Part model, mm, in its own coordinate system. Face numbers are marked on the shaded views. A direction names the side the tool comes from. Round coordinates to 2 decimals unless told otherwise and drop trailing zeros. Loops run counter-clockwise (first coordinate to the right, second up) from the corner with the lowest first, then second, coordinate; pieces in that order, holes last. Notation, with made-up numbers: (46, 4) - (94, 4) arc R27 cw to (94, 20) - close; hole circle Ø5 at (74, 62). An arc over 180 degrees is marked (long way). Put each result on its own line as item: value.
from build123d import *

# Parameters (mm, degrees)
SKETCH3_R               = 9
EXTRUDE2_DEPTH          = 28.5
EXTRUDE2_DEPTH_BACK     = 28.5
SKETCH4_R               = 9
SKETCH4_R_2             = 7.8
CUT_EXTRUDE2_DEPTH      = 26.5
CUT_EXTRUDE2_DEPTH_BACK = 26.5
SKETCH5_R               = 3.5
EXTRUDE3_DEPTH          = 48.5
EXTRUDE3_DEPTH_BACK     = 48.5


with BuildPart() as part:
    # Sketch3 → Extrude2 (new body, two sides)
    with BuildSketch(Plane(origin=(0, 0, 0), x_dir=(1, 0, 0), z_dir=(0, 1, 0))) as extrude2_sk:
        Circle(SKETCH3_R)
    extrude(amount=EXTRUDE2_DEPTH)
    extrude(extrude2_sk.sketch, amount=-EXTRUDE2_DEPTH_BACK)

    # Sketch4 → Cut-Extrude2 (cut, two sides)
    with BuildSketch(Plane(origin=(0, 0, 0), x_dir=(1, 0, 0), z_dir=(0, 1, 0))) as cut_extrude2_sk:
        Circle(SKETCH4_R)
        Circle(SKETCH4_R_2, mode=Mode.SUBTRACT)
    extrude(amount=CUT_EXTRUDE2_DEPTH, mode=Mode.SUBTRACT)
    extrude(cut_extrude2_sk.sketch, amount=-CUT_EXTRUDE2_DEPTH_BACK, mode=Mode.SUBTRACT)

    # Sketch5 → Extrude3 (add, two sides)
    with BuildSketch(Plane(origin=(0, 0, 0), x_dir=(1, 0, 0), z_dir=(0, 1, 0))) as extrude3_sk:
        Circle(SKETCH5_R)
    extrude(amount=EXTRUDE3_DEPTH)
    extrude(extrude3_sk.sketch, amount=-EXTRUDE3_DEPTH_BACK)


solid = part.part
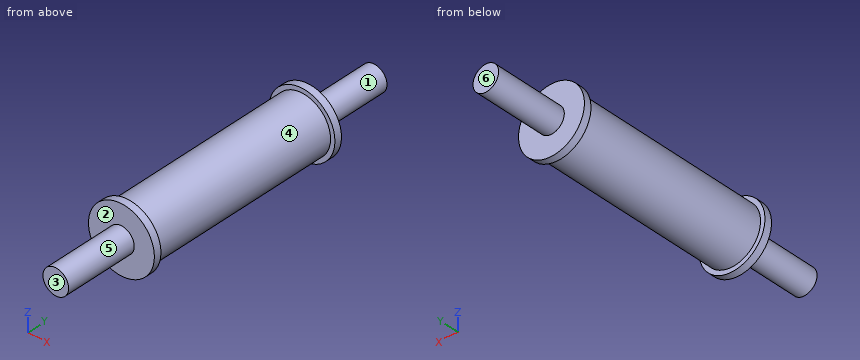
1. Probe line 1 along Y through (x, z) = (7, 5.25); line 2 along Y through (x, z) = (0.5, -4.75); line 3 along Z through (x, y) = (0, 36.5). List the from-to ranges inside material, lowest first. Write a range as [from, to].
A:
line 1: y = [-28.5, -26.5], [26.5, 28.5]
line 2: y = [-28.5, 28.5]
line 3: z = [-3.5, 3.5]
2. Band-saw the part on D-D (x = -5.25). List the corners of the cut face in (y, z).
A:
outline: (-28.5, -7.31) - (-26.5, -7.31) - (-26.5, -5.77) - (26.5, -5.77) - (26.5, -7.31) - (28.5, -7.31) - (28.5, 7.31) - (26.5, 7.31) - (26.5, 5.77) - (-26.5, 5.77) - (-26.5, 7.31) - (-28.5, 7.31) - close
3. Two-plate mould, pull along Y, no slides. Class the marked faces 3, 4, 5 and 6: pulls with the +Y half, pulls with the -Y half, needs draft (parallel to the pull), parting line crosses it, or undercut.
A:
face 3: pulls with the -Y half
face 4: undercut
face 5: needs draft
face 6: pulls with the +Y half
4. Band-saw the part on B-B (z = 0). List the corners of the cut face in (x, y), plus the area to 3 significant figures.
A:
outline: (-9, -28.5) - (-3.5, -28.5) - (-3.5, -48.5) - (3.5, -48.5) - (3.5, -28.5) - (9, -28.5) - (9, -26.5) - (7.8, -26.5) - (7.8, 26.5) - (9, 26.5) - (9, 28.5) - (3.5, 28.5) - (3.5, 48.5) - (-3.5, 48.5) - (-3.5, 28.5) - (-9, 28.5) - (-9, 26.5) - (-7.8, 26.5) - (-7.8, -26.5) - (-9, -26.5) - close
area: 1,180 mm²
5. Band-saw the part on A-A (x = 0). List the corners of the cut face in (y, z).
A:
outline: (-48.5, -3.5) - (-28.5, -3.5) - (-28.5, -9) - (-26.5, -9) - (-26.5, -7.8) - (26.5, -7.8) - (26.5, -9) - (28.5, -9) - (28.5, -3.5) - (48.5, -3.5) - (48.5, 3.5) - (28.5, 3.5) - (28.5, 9) - (26.5, 9) - (26.5, 7.8) - (-26.5, 7.8) - (-26.5, 9) - (-28.5, 9) - (-28.5, 3.5) - (-48.5, 3.5) - close
6. Pin check, flat tips, straight feed: P1, Ø3, axis at x = -4.5, y = 2.5, coming from the -Z side; P2, Ø4, axis at x = 2.5, y = 29, coming from the +Z side; P3, Ø4, axis at y = -11, z = 7, coming from the +X side. Stop position of each tip, or through.
A:
P1: stops at z = -7.2
P2: stops at z = 8.98
P3: stops at x = 5.99
7. Tool access for the marked faces 1 and 2: list every direction of +Z, -Z, +X, -X, +Y, -Y with a clear straight run to the whole face (end or side of a thin tool).
A:
face 1: +Y
face 2: -Y
8. Band-saw the part on C-C (y = -18.5). List the corners of the cut face in (x, z).
A:
outline: circle Ø15.6 at (0, 0)
